```python
from build123d import *

# Parameters (mm, degrees)
BOSS_EXTRUDE3_DEPTH  = 6.55
BOSS_EXTRUDE4_DEPTH  = 15
BOSS_EXTRUDE5_START  = 2
SKETCH1_4_R          = 1.5
BOSS_EXTRUDE5_DEPTH  = 4.55
BOSS_EXTRUDE6_START  = -6.55
SKETCH1_6_R          = 1.5
BOSS_EXTRUDE6_DEPTH  = 4.55
SKETCH1_8_R          = 1.5
BOSS_EXTRUDE11_DEPTH = 2.55
BOSS_EXTRUDE12_START = -13.75
BOSS_EXTRUDE12_DEPTH = 3.471884434
BOSS_EXTRUDE13_START = -13.75
SKETCH4_6_R          = 1
BOSS_EXTRUDE13_DEPTH = 13.75
BOSS_EXTRUDE14_START = -13.75
SKETCH4_7_R          = 1
BOSS_EXTRUDE14_DEPTH = 4
BOSS_EXTRUDE15_START = -16.75
BOSS_EXTRUDE15_DEPTH = 1
BOSS_EXTRUDE16_START = -13.75
BOSS_EXTRUDE16_DEPTH = 1.2


# Read off the part's stored shape, not the designer's step: Boss-Extrude12
with BuildPart() as part:
    # Sketch1 → Boss-Extrude3 (new, symmetric)
    with BuildSketch(Plane(origin=(0, 0, 0), x_dir=(1, 0, 0), z_dir=(0, 1, 0))):
        with BuildLine():
            Line((-2.040057994, 14.503003078), (-13.75, 0))
            Line((-13.75, 0), (-6.875, 0))
            Line((-6.875, 0), (0, 0))
            Line((0, 0), (2, 0))
            Line((2, 0), (2, 15))
            Line((2, 15), (-1, 15))
            ThreePointArc((-1, 15), (-1.576352013, 14.869367868), (-2.040057994, 14.503003078))
        make_face()
    extrude(amount=BOSS_EXTRUDE3_DEPTH, both=True)

    # Sketch2 → Boss-Extrude4 (add)
    with BuildSketch(Plane(origin=(0, 0, -15), x_dir=(-1, 0, 0), z_dir=(0, 0, -1))):
        Polygon((-2, 6.55), (-5.781644263, 0), (-2, -6.55), align=None)
    extrude(amount=-BOSS_EXTRUDE4_DEPTH)

    # Sketch1<4> → Boss-Extrude5 (add)
    with BuildSketch(Plane(origin=(0, 0, 0), x_dir=(1, 0, 0), z_dir=(0, 1, 0)).offset(BOSS_EXTRUDE5_START)):
        with BuildLine():
            Line((-6.875, 0), (-13.75, 0))
            Line((-13.75, 0), (-13.75, -3))
            ThreePointArc((-13.75, -3), (-10.75, -6), (-7.75, -3))
            Line((-7.75, -3), (-7.75, -0.875))
            ThreePointArc((-7.75, -0.875), (-7.493718434, -0.256281566), (-6.875, 0))
        make_face()
        with Locations(Location((-10.75, -3, 0), (0, 0, 270))):
            Circle(SKETCH1_4_R, mode=Mode.SUBTRACT)
    extrude(amount=BOSS_EXTRUDE5_DEPTH)

    # Sketch1<6> → Boss-Extrude6 (add)
    with BuildSketch(Plane(origin=(0, 0, 0), x_dir=(1, 0, 0), z_dir=(0, 1, 0)).offset(BOSS_EXTRUDE6_START)):
        with BuildLine():
            Line((-6.875, 0), (-13.75, 0))
            Line((-13.75, 0), (-13.75, -3))
            ThreePointArc((-13.75, -3), (-10.75, -6), (-7.75, -3))
            Line((-7.75, -3), (-7.75, -0.875))
            ThreePointArc((-7.75, -0.875), (-7.493718434, -0.256281566), (-6.875, 0))
        make_face()
        with Locations(Location((-10.75, -3, 0), (0, 0, 270))):
            Circle(SKETCH1_6_R, mode=Mode.SUBTRACT)
    extrude(amount=BOSS_EXTRUDE6_DEPTH)

    # Sketch1<8> → Boss-Extrude11 (add, symmetric)
    with BuildSketch(Plane(origin=(0, 0, 0), x_dir=(1, 0, 0), z_dir=(0, 1, 0))):
        with BuildLine():
            Line((0, 0), (-6.875, 0))
            ThreePointArc((-6.875, 0), (-6.256281566, -0.256281566), (-6, -0.875))
            Line((-6, -0.875), (-6, -3))
            ThreePointArc((-6, -3), (-3, -6), (0, -3))
            Line((0, -3), (0, 0))
        make_face()
        with Locations(Location((-3, -3, 0), (0, 0, 270))):
            Circle(SKETCH1_8_R, mode=Mode.SUBTRACT)
    extrude(amount=BOSS_EXTRUDE11_DEPTH, both=True)

    # Boss-Extrude12 outline → Boss-Extrude12 (add)
    with BuildSketch(Plane(origin=(0, 0, 0), x_dir=(0, 0, -1), z_dir=(1, 0, 0)).offset(BOSS_EXTRUDE12_START)):
        with BuildLine():
            Line((3.4, 1), (0, 1))
            Line((0, 1), (0, -1))
            Line((0, -1), (3.4, -1))
            ThreePointArc((3.4, -1), (4.036396103, -0.736396103), (4.3, -0.1))
            Line((4.3, -0.1), (4.3, 0.1))
            ThreePointArc((4.3, 0.1), (4.036396103, 0.736396103), (3.4, 1))
        make_face()
    extrude(amount=BOSS_EXTRUDE12_DEPTH)

    # Sketch4<6> → Boss-Extrude13 (add)
    with BuildSketch(Plane(origin=(0, 0, 0), x_dir=(0, 0, -1), z_dir=(1, 0, 0)).offset(BOSS_EXTRUDE13_START)):
        with Locations((2.6, 0)):
            Circle(SKETCH4_6_R)
        with BuildLine():
            Line((2.6, -1), (0, -1))
            ThreePointArc((0, -1), (5.385677655, 0), (0, 1))
            Line((0, 1), (2.6, 1))
            Line((2.6, 1), (3.4, 1))
            ThreePointArc((3.4, 1), (4.036396103, 0.736396103), (4.3, 0.1))
            Line((4.3, 0.1), (4.3, -0.1))
            ThreePointArc((4.3, -0.1), (4.036396103, -0.736396103), (3.4, -1))
            Line((3.4, -1), (2.6, -1))
        make_face()
    extrude(amount=BOSS_EXTRUDE13_DEPTH)

    # Sketch4<7> → Boss-Extrude14 (add)
    with BuildSketch(Plane(origin=(0, 0, 0), x_dir=(0, 0, -1), z_dir=(1, 0, 0)).offset(BOSS_EXTRUDE14_START)):
        with Locations((2.6, 0)):
            Circle(SKETCH4_7_R)
    extrude(amount=-BOSS_EXTRUDE14_DEPTH)

    # Sketch4<8> → Boss-Extrude15 (add)
    with BuildSketch(Plane(origin=(0, 0, 0), x_dir=(0, 0, -1), z_dir=(1, 0, 0)).offset(BOSS_EXTRUDE15_START)):
        with BuildLine():
            ThreePointArc((3.6, 0), (3.307106781, -0.707106781), (2.6, -1))
            Line((2.6, -1), (3.4, -1))
            ThreePointArc((3.4, -1), (4.036396103, -0.736396103), (4.3, -0.1))
            Line((4.3, -0.1), (4.3, 0.1))
            ThreePointArc((4.3, 0.1), (4.036396103, 0.736396103), (3.4, 1))
            Line((3.4, 1), (2.6, 1))
            ThreePointArc((2.6, 1), (3.307106781, 0.707106781), (3.6, 0))
        make_face()
    extrude(amount=-BOSS_EXTRUDE15_DEPTH)

    # Sketch4<9> → Boss-Extrude16 (add)
    with BuildSketch(Plane(origin=(0, 0, 0), x_dir=(0, 0, -1), z_dir=(1, 0, 0)).offset(BOSS_EXTRUDE16_START)):
        with BuildLine():
            Line((0, -1), (2.6, -1))
            ThreePointArc((2.6, -1), (1.6, 0), (2.6, 1))
            Line((2.6, 1), (0, 1))
            Line((0, 1), (0, -1))
        make_face()
    extrude(amount=-BOSS_EXTRUDE16_DEPTH)


solid = part.part
```
Here's how the part is built. I have some questions about the finished solid (model axes, mm). A direction names the side the tool comes from. Round coordinates to 2 decimals unless told otherwise and drop trailing zeros. Write each loop counter-clockwise with the first axis right and the second up, starting at its lowest first coordinate (ties: lowest second). Pieces come first, ordered by that corner, then holes. Notation, with made-up numbers: M -6,89 L 4,89 A28 cw 4,110 Z; hole C -24,-27 d5. An arc over 180 degrees is marked long. Answer as CSV lines item,"result". Start each with the question number.
1. Suppose I cut it at D-D on x = -3. Write out the boundary of the cut face in (y, z).
2. On a 3-axis mill with a long thin cutter (end or side, diameter ignored), from which of +Z, -Z, +X, -X, +Y, -Y can I reach the whole of each face in a straight line? I mean faces 1 (the flat face through (-2, 2.55, 1.6)), 2 (the flat face through (-6, 0, 2)), 3 (the cylindrical face through (-17.24, 0.73, -4.04)), 4 (the flat face through (-14, -1, -1)). Say none if no direction works.
3. Suppose I cut it at B-B on z = 0.5. Write out the boundary of the cut face in (x, y), then the cut area to 3 significant figures.
4. Suppose I cut it at C-C on y = 5.25. Write out the boundary of the cut face in (x, z) (3 decimals), then the cut area to 3 significant figures.
5. Thinking about a two-plate mould opening in Z: for faces 5 (the flat face through (-16.75, 0, -4)), 6 (the flat face through (2, 0, -15)), 7 (the cylindrical face through (-12.08, 4.24, 3.69)), which applies, released by +Z, released by -Z, zero draft, split by the parting line, or undercut?
6. Suppose I cut it at A-A on x = -10.75. Write out the boundary of the cut face in (y, z), then the cut area to 3 significant figures.
7. I need wall thicknesses on probe 1 along Y at (x, z) = (-13.5, 1.5); probe 2 along X at (y, z) = (1.45, 3); probe 3 along X at (y, z) = (-3.3, 3). Which ranges of each line are inside material? Lowest first, please.
8. I'm going to push flat-ended pins straight in: pin 1 Ø0.6 at (y, z) = (-5, 2.5) entering from +X; pin 2 Ø1.5 at (y, z) = (-4, 1) entering from -X; pin 3 Ø5 at (y, z) = (-1, -2.5) entering from +X. Where does each tip first touch, or does it pass through?
Check result:
1,outline,"M -6.55,-13.31 L 6.55,-13.31 L 6.55,0 L 2.55,0 L 2.55,1.5 L -2.55,1.5 L -2.55,0 L -6.55,0 Z; M -2.55,4.5 L 2.55,4.5 L 2.55,6 L -2.55,6 Z"
2,face 1,"+Z, +X, +Y"
2,face 2,"+Z, +Y, -Y"
2,face 3,"-Z, -X, +Y"
2,face 4,"+Z, -Z, -X, -Y"
3,outline,"M -13.75,-6.55 L -7.67,-6.55 L -7.67,-2 L -13.75,-2 Z; M -13.75,2 L -7.67,2 L -7.67,6.55 L -13.75,6.55 Z; M -6.08,-2.55 L 0,-2.55 L 0,2.55 L -6.08,2.55 Z"
3,area,"86.4 mm2"
4,outline,"M -13.75,0 L -2.04,-14.503 A1.337 ccw -1,-15 L 2.751,-15 L 2.751,0 L -6.875,0 A0.875 cw -7.75,0.875 L -7.75,3 A3 ccw -13.75,3 Z; hole C -10.75,3 d3"
4,area,"182 mm2"
5,face 5,"zero draft"
5,face 6,"released by -Z"
5,face 7,"undercut"
6,outline,"M -6.55,-3.72 L -2.55,-3.72 A2.79 ccw 2.55,-3.72 L 6.55,-3.72 L 6.55,1.5 L 2,1.5 L 2,0 L -2,0 L -2,1.5 L -6.55,1.5 Z; M -6.55,4.5 L -2,4.5 L -2,6 L -6.55,6 Z; M 2,4.5 L 6.55,4.5 L 6.55,6 L 2,6 Z"
6,area,"82.1 mm2"
7,probe 1,"y = -6.55 to -2, 2 to 6.55"
7,probe 2,"x = -6 to -4.5, -1.5 to 0"
7,probe 3,"x = -13.75 to -12.25, -9.25 to -7.75"
8,pin 1,"stops at x = -7.75"
8,pin 2,"stops at x = -13.75"
8,pin 3,"stops at x = 5.78"
